```python
from build123d import *

# Parameters (mm, degrees)
F0_W     = 15
F0_H     = 60
F1_DEPTH = 28.5
F3_W     = 56.5
F3_H     = 50
F4_DEPTH = 28.501
F2_W     = 15
F2_H     = 21.875
F5_DEPTH = 12.25
F6_DEPTH = 71.5
F7_DEPTH = 40.751
F8_DEPTH = 0.66


with BuildPart() as f1:
    # F0 (on Top) → F1 (new body)
    with BuildSketch(Plane.XY):
        Rectangle(F0_W, F0_H)
    extrude(amount=F1_DEPTH)

    # F3 (on face) → F4 (cut, through all)
    with BuildSketch(Plane(origin=(0, 0, 0), x_dir=(1, 0, 0), z_dir=(0, 0, -1))):
        with Locations((35.75, -5)):
            Rectangle(F3_W, F3_H)
    extrude(amount=-F4_DEPTH, mode=Mode.SUBTRACT)

    # F2 (on face) → F5 (join)
    with BuildSketch(Plane.XY.offset(28.5)):
        with Locations((0, 19.0625)):
            Rectangle(F2_W, F2_H)
        with Locations((0, -19.0625)):
            Rectangle(F2_W, F2_H)
    extrude(amount=F5_DEPTH)

    # F6 (add): a face of the model
    f6_faces = [f1.faces().sort_by_distance(p)[0] for p in [
        (7.5, 0, 19.1119903993),
    ]]
    extrude(f6_faces, amount=F6_DEPTH)

    # F3 (on face) → F7 (cut, through all)
    with BuildSketch(Plane(origin=(0, 0, 0), x_dir=(1, 0, 0), z_dir=(0, 0, -1))):
        with Locations((35.75, -5)):
            Rectangle(F3_W, F3_H)
    extrude(amount=-F7_DEPTH, mode=Mode.SUBTRACT)

    # F8 (cut): faces of the model
    f8_faces = [f1.faces().sort_by_distance(p)[0] for p in [
        (0, 0, 28.5),
        (71.5, 0, 28.5),
    ]]
    extrude(f8_faces, amount=-F8_DEPTH, mode=Mode.SUBTRACT)


solid = f1.part
```
Verification items for the finished model (mm, model axes). A direction names the side the tool comes from. Round coordinates to 2 decimals unless told otherwise and drop trailing zeros. Write each loop counter-clockwise with the first axis right and the second up, starting at its lowest first coordinate (ties: lowest second). Pieces come first, ordered by that corner, then holes. Notation, with made-up numbers: (38, 81) -> (83, 81) arc R12 cw to (83, 89) -> close; hole circle Ø10 at (52, -16). An arc over 180 degrees is marked (long way). Write each question's results on one line, items separated by ' | '.
Q1. Sectioned sample at C-C, the plane z = 6. Record the boundary of the cut face in (x, y), and give its area (4 significant figures).
Derived:
outline: (-7.5, -30) -> (79, -30) -> (79, 30) -> (64, 30) -> (64, -20) -> (7.5, -20) -> (7.5, 30) -> (-7.5, 30) -> close | area: 2,365 mm²
Q2. Draft check along X on faces 4 (the face through (0, 19, 40.75)), 5 (the face through (79, 0, 20)), 6 (the face through (-7.5, 0, 20)), 7 (the face through (35, -20, 20)). Enter one of: released by +X, released by -X, zero draft, split by the parting line, or undercut.
Derived:
face 4: zero draft | face 5: released by +X | face 6: released by -X | face 7: undercut
Q3. Sectioned sample at A-A, the plane y = -1. Record the boundary of the cut face in (x, z).
Derived:
outline: (-7.5, 0) -> (7.5, 0) -> (7.5, 27.84) -> (-7.5, 27.84) -> close; (64, 0) -> (79, 0) -> (79, 27.84) -> (64, 27.84) -> close
Q4. Access from +Z, -Z, +X, -X, +Y, -Y to the whole of each face (thin tool, end or side, straight path). Record for faces 1 (the face through (64, 5, 20)), 2 (the face through (0, 30, 21)), 3 (the face through (0, 0, 27.84)).
Derived:
face 1: +Z, -Z, +Y | face 2: +Z, -Z, +X, -X, +Y | face 3: +Z, +X, -X
Q5. Go/stop test with flat-tipped pins: pin 1 Ø12 at (x, y) = (1, 0.5) entering from +Z; pin 2 Ø1.5 at (x, z) = (16.5, 15) entering from +Y. Record where each tip stops, or that it passes through.
Derived:
pin 1: stops at z = 27.84 | pin 2: stops at y = -20
Q6. Sectioned sample at D-D, the plane x = 71.5. Record the boundary of the cut face in (y, z) (3 decimals).
Derived:
outline: (-30, 0) -> (30, 0) -> (30, 40.75) -> (8.125, 40.75) -> (8.125, 27.84) -> (-8.125, 27.84) -> (-8.125, 40.75) -> (-30, 40.75) -> close
Q7. Sectioned sample at B-B, the plane z = 35. Record the boundary of the cut face in (x, y) (3 decimals), and give its area (3 significant figures).
Derived:
outline: (-7.5, -30) -> (79, -30) -> (79, -8.125) -> (64, -8.125) -> (64, -20) -> (7.5, -20) -> (7.5, -8.125) -> (-7.5, -8.125) -> close; (-7.5, 8.125) -> (7.5, 8.125) -> (7.5, 30) -> (-7.5, 30) -> close; (64, 8.125) -> (79, 8.125) -> (79, 30) -> (64, 30) -> close | area: 1,880 mm²
Q8. Thickness scan on probe 1 along X at (y, z) = (12.5, 36.5); probe 2 along Y at (x, z) = (8, 18); probe 3 along Z at (x, y) = (4, -6.5). Record the ranges inside material, lowest first.
Derived:
probe 1: x = -7.5 to 7.5, 64 to 79 | probe 2: y = -30 to -20 | probe 3: z = 0 to 27.84
